```python
from build123d import *

# Parameters (mm, degrees)
SKIZZE1_W                       = 32
SKIZZE1_H                       = 44.5
AUFSATZ_LINEAR_AUSTRAGEN1_DEPTH = 3
AUFSATZ_LINEAR_AUSTRAGEN2_DEPTH = 32
SKIZZE3_R                       = 12.5
SCHNITT_LINEAR_AUSTRAGEN1_DEPTH = 57.879609703
VERRUNDUNG1_R                   = 4
VERRUNDUNG2_R                   = 4


with BuildPart() as part:
    # Skizze1 → Aufsatz-Linear austragen1 (new body)
    with BuildSketch(Plane.XY):
        with Locations((16, 22.25)):
            Rectangle(SKIZZE1_W, SKIZZE1_H)
    extrude(amount=AUFSATZ_LINEAR_AUSTRAGEN1_DEPTH)

    # Skizze2 → Aufsatz-Linear austragen2 (add, through all)
    with BuildSketch(Plane(origin=(32, 0, 0), x_dir=(0, 0, -1), z_dir=(1, 0, 0))):
        with BuildLine():
            Line((0, 44.5), (15.2, 44.5))
            Line((15.2, 44.5), (15.2, 38.5))
            Line((15.2, 38.5), (12.2, 38.5))
            Line((12.2, 38.5), (12.2, 40.6))
            ThreePointArc((12.2, 40.6), (11.936396103, 41.236396103), (11.3, 41.5))
            Line((11.3, 41.5), (10.9, 41.5))
            ThreePointArc((10.9, 41.5), (10.263603897, 41.236396103), (10, 40.6))
            Line((10, 40.6), (10, 38.5))
            Line((10, 38.5), (-3, 38.5))
            Line((-3, 38.5), (-3, 44.5))
            Line((-3, 44.5), (0, 44.5))
        make_face()
        with BuildLine():
            Line((0, 0), (-3, 0))
            Line((-3, 0), (-3, 6))
            Line((-3, 6), (10, 6))
            Line((10, 6), (10, 3.9))
            ThreePointArc((10, 3.9), (10.263603897, 3.263603897), (10.9, 3))
            Line((10.9, 3), (11.3, 3))
            ThreePointArc((11.3, 3), (11.936396103, 3.263603897), (12.2, 3.9))
            Line((12.2, 3.9), (12.2, 6))
            Line((12.2, 6), (15.2, 6))
            Line((15.2, 6), (15.2, 0))
            Line((15.2, 0), (0, 0))
        make_face()
    extrude(amount=-AUFSATZ_LINEAR_AUSTRAGEN2_DEPTH)

    # Skizze3 → Schnitt-Linear austragen1 (cut, through all)
    with BuildSketch(Plane(origin=(0, 0, 0), x_dir=(-1, 0, 0), z_dir=(0, 0, -1))):
        with Locations((-16, 22.25)):
            Circle(SKIZZE3_R)
    extrude(amount=-SCHNITT_LINEAR_AUSTRAGEN1_DEPTH, mode=Mode.SUBTRACT)

    # Verrundung1
    verrundung1_edges = [part.edges().sort_by_distance(p)[0] for p in [
        (16, 44.5, 3),
        (16, 0, 3),
    ]]
    fillet(verrundung1_edges, radius=VERRUNDUNG1_R)

    # Verrundung2
    verrundung2_edges = [part.edges().sort_by_distance(p)[0] for p in [
        (16, 44.5, -15.2),
        (16, 0, -15.2),
    ]]
    fillet(verrundung2_edges, radius=VERRUNDUNG2_R)


solid = part.part
```
Source: CAD feature listing. Evaluate the final solid. Frame: model axes, mm. A direction names the side the tool comes from. Coordinates: 2 decimals unless noted, no trailing zeros. Write each loop counter-clockwise with the first axis right and the second up, starting at its lowest first coordinate (ties: lowest second). Pieces come first, ordered by that corner, then holes. Notation, with made-up numbers: (37.25, 53) -> (55.25, 53) arc R34 ccw to (55.25, 88) -> close; hole circle Ø6 at (67.25, 25.25). An arc over 180 degrees is marked (long way). Return JSON: item names as keys, results as strings. Group by question number.
1) Mould query, pull axis Z, two halves, no side actions, for faces 4 (the face through (15.776, 1.141, -13.997)), 5 (the face through (16, 5, -12.2)), 6 (the face through (16, 6, -14)), 7 (the face through (16, 40, -12.2)). Classes: +Z half, -Z half, draft (parallel to the pull), parting line (faces both ways), or undercut.
2) Section query B-B, the plane y = 22.25. Return loops of the section in (x, z), plus the area to 3 significant figures.
3) Ray query, line 1 along Z through (x, y) = (15, 4); line 2 along Y through (x, z) = (24, -9); line 3 along Z through (x, y) = (9.5, 33). Return the intervals inside material, ascending.
4) Section query A-A, the plane x = 4. Return loops of the section in (y, z), plus the area to 3 significant figures.
5) Set-up query: faces 1 (the face through (16, 38.5, -5)), 2 (the face through (16, 44.5, -6)), 3 (the face through (16.22, 41.24, -10.27)). Return all of +Z, -Z, +X, -X, +Y, -Y with unobstructed straight access to the full face (end or side cutting, diameter ignored); none if empty.
6) Contact query for flat-ended pins moving along their axis: P1, Ø6, axis at y = 33.5, z = -13, coming from the +X side; P2, Ø2, axis at y = 39.5, z = -2.5, coming from the -X side; P3, Ø1.5, axis at x = 20.5, z = -13.5, coming from the +Y side; P4, Ø16, axis at x = 21, y = 26.5, coming from the -Z side. Output: stop coordinate, or through.
7) Section query D-D, the plane x = 16. Return loops of the section in (y, z).
8) Section query C-C, the plane z = -6.75. Return loops of the section in (x, y).
From the geometry:
{
 "1": {"face 4": "-Z half", "face 5": "undercut", "face 6": "draft", "face 7": "undercut"},
 "2": {"outline": "(0, 0) -> (3.5, 0) -> (3.5, 3) -> (0, 3) -> close; (28.5, 0) -> (32, 0) -> (32, 3) -> (28.5, 3) -> close", "area": "21.0 mm²"},
 "3": {"line 1": "-15.2 to -12.2, -10 to 3", "line 2": "0 to 6, 38.5 to 44.5", "line 3": "0 to 3"},
 "4": {"outline": "(0, -11.2) arc R4 ccw to (4, -15.2) -> (6, -15.2) -> (6, -12.2) -> (3.9, -12.2) arc R0.9 cw to (3, -11.3) -> (3, -10.9) arc R0.9 cw to (3.9, -10) -> (6, -10) -> (6, 0) -> (18.75, 0) -> (18.75, 3) -> (4, 3) arc R4 ccw to (0, -1) -> close; (25.75, 0) -> (38.5, 0) -> (38.5, -10) -> (40.6, -10) arc R0.9 cw to (41.5, -10.9) -> (41.5, -11.3) arc R0.9 cw to (40.6, -12.2) -> (38.5, -12.2) -> (38.5, -15.2) -> (40.5, -15.2) arc R4 ccw to (44.5, -11.2) -> (44.5, -1) arc R4 ccw to (40.5, 3) -> (25.75, 3) -> close", "area": "269 mm²"},
 "5": {"face 1": "-Z, +X, -X", "face 2": "+Z, -Z, +X, -X, +Y", "face 3": "+X, -X"},
 "6": {"P1": "through", "P2": "x = 0", "P3": "y = 44.19", "P4": "z = 0"},
 "7": {"outline": "(0, -11.2) arc R4 ccw to (4, -15.2) -> (6, -15.2) -> (6, -12.2) -> (3.9, -12.2) arc R0.9 cw to (3, -11.3) -> (3, -10.9) arc R0.9 cw to (3.9, -10) -> (6, -10) -> (6, 0) -> (9.75, 0) -> (9.75, 3) -> (4, 3) arc R4 ccw to (0, -1) -> close; (34.75, 0) -> (38.5, 0) -> (38.5, -10) -> (40.6, -10) arc R0.9 cw to (41.5, -10.9) -> (41.5, -11.3) arc R0.9 cw to (40.6, -12.2) -> (38.5, -12.2) -> (38.5, -15.2) -> (40.5, -15.2) arc R4 ccw to (44.5, -11.2) -> (44.5, -1) arc R4 ccw to (40.5, 3) -> (34.75, 3) -> close"},
 "8": {"outline": "(0, 0) -> (32, 0) -> (32, 6) -> (0, 6) -> close; (0, 38.5) -> (32, 38.5) -> (32, 44.5) -> (0, 44.5) -> close"}
}
